Source: CAD feature listing. Evaluate the final solid. Frame: model axes, mm. Coordinates: 2 decimals unless noted, no trailing zeros. Write each loop counter-clockwise with the first axis right and the second up, starting at its lowest first coordinate (ties: lowest second). Pieces come first, ordered by that corner, then holes. Notation, with made-up numbers: (-32, -33.75) -> (18, -33.75) arc R15 cw to (18, -15.75) -> close; hole circle Ø1 at (-25.5, -32.5). An arc over 180 degrees is marked (long way). One line per item, written item: value. Start each with the question number.
1. Section query D-D, the plane x = 62.5. Output: boundary loops of the cut face in (y, z), and give its area (3 significant figures).
2. Section query C-C, the plane x = 58. Output: boundary loops of the cut face in (y, z), and give its area (3 significant figures).
3. Mould query, pull axis Z, two halves, no side actions, for faces 1 (the flat face through (54.8, -2.9, -7)), 2 (the flat face through (55, 0, 0)), 3 (the cylindrical face through (61.867, -2.962, -0.128)). Classes: released by +Z, released by -Z, zero draft, split by the parting line, or undercut.
4. Section query A-A, the plane y = -3.75. Output: boundary loops of the cut face in (x, z).
5. Section query B-B, the plane z = 0. Output: boundary loops of the cut face in (x, y).
6. First-contact query: P1, Ø4.5, axis at x = 58.95, z = 0, coming from the -Y side (1 decimal); P2, Ø2, axis at x = 64, y = -3.5, coming from the +Z side; P3, Ø2, axis at x = 54, y = -2.5, coming from the -Z side. Flat tips, straight axial feed; report the tip coordinate or a pass-through.
7. Line query: line 1 (X direction, y = -3.75, z = -1.25); line 2 (Z direction, x = 58.25, y = -1.35); line 3 (Z direction, x = 57.5, y = -1.3). Output: solid intervals per line, ascending.
from build123d import *

# Parameters (mm, degrees)
F1_DEPTH = 5.842
F2_D     = 5.842


# Not quite as in the source:
# - a feature names something its author has since deleted; it is built from what else it names


with BuildPart() as f1:
    # F0 (on Front) → F1 (new body)
    with BuildSketch(Plane.XZ):
        Polygon((58.9488451577, 9.395414032), (50.8121779269, 4.697707016), (50.8121779269, -4.697707016), (58.9488451577, -9.395414032), (67.0855123886, -4.697707016), (67.0855123886, 4.697707016), align=None)
    extrude(amount=F1_DEPTH)

    # F2 (through all)
    with Locations(Plane(origin=(0, 0, 0), x_dir=(1, 0, 0), z_dir=(0, 1, 0))):
        with Locations((58.9488451577, 0)):
            Hole(F2_D / 2)


solid = f1.part
Computed values:
1. outline: (-5.84, -7.35) -> (0, -7.35) -> (0, 7.35) -> (-5.84, 7.35) -> close
1. area: 85.8 mm²
2. outline: (-5.84, -8.85) -> (0, -8.85) -> (0, -2.76) -> (-5.84, -2.76) -> close; (-5.84, 2.76) -> (0, 2.76) -> (0, 8.85) -> (-5.84, 8.85) -> close
2. area: 71.1 mm²
3. face 1: released by -Z
3. face 2: zero draft
3. face 3: undercut
4. outline: (50.81, -4.7) -> (58.95, -9.4) -> (67.09, -4.7) -> (67.09, 4.7) -> (58.95, 9.4) -> (50.81, 4.7) -> close; hole circle Ø5.84 at (58.95, 0)
5. outline: (50.81, -5.84) -> (56.03, -5.84) -> (56.03, 0) -> (50.81, 0) -> close; (61.87, -5.84) -> (67.09, -5.84) -> (67.09, 0) -> (61.87, 0) -> close
6. P1: passes through
6. P2: stops at z = 7.06
6. P3: stops at z = -7.12
7. line 1: x = 50.81 to 56.31, 61.59 to 67.09
7. line 2: z = -8.99 to -2.84, 2.84 to 8.99
7. line 3: z = -8.56 to -2.54, 2.54 to 8.56
